Here's how the part is built. I have some questions about the finished solid (model axes, mm). Give positions to 0.01 mm unless a question says otherwise; leave off trailing zeros. Loops run counter-clockwise (first coordinate to the right, second up) from the corner with the lowest first, then second, coordinate; pieces in that order, holes last. Notation, with made-up numbers: (80.25, 12) - (90.25, 12) arc R17 cw to (90.25, 41) - close; hole circle Ø6 at (-6.75, -11). An arc over 180 degrees is marked (long way). Use a Markdown table: item, result.
from build123d import *

# Parameters (mm, degrees)
SKETCH1_R           = 25
BOSS_EXTRUDE1_DEPTH = 3
SKETCH4_R           = 12.5
CUT_EXTRUDE1_DEPTH  = 8.2
SKETCH11_R          = 2
CUT_EXTRUDE2_DEPTH  = 10


with BuildPart() as part:
    # Sketch1 → Boss-Extrude1 (new body)
    with BuildSketch(Plane.XY):
        Circle(SKETCH1_R)
    extrude(amount=BOSS_EXTRUDE1_DEPTH)

    # Sketch4 → Cut-Extrude1 (cut)
    with BuildSketch(Plane(origin=(0, 0, 0), x_dir=(-1, 0, 0), z_dir=(0, 0, -1))):
        Circle(SKETCH4_R)
    extrude(amount=-CUT_EXTRUDE1_DEPTH, mode=Mode.SUBTRACT)

    # Sketch11 → Cut-Extrude2 (cut)
    with BuildSketch(Plane(origin=(0, 0, 0), x_dir=(-1, 0, 0), z_dir=(0, 0, -1))):
        with Locations((0, 18.75)):
            Circle(SKETCH11_R)
        with Locations((16.237976321, 9.375)):
            Circle(SKETCH11_R)
        with Locations((16.237976321, -9.375)):
            Circle(SKETCH11_R)
        with Locations((0, -18.75)):
            Circle(SKETCH11_R)
        with Locations((-16.237976321, -9.375)):
            Circle(SKETCH11_R)
        with Locations((-16.237976321, 9.375)):
            Circle(SKETCH11_R)
    extrude(amount=-CUT_EXTRUDE2_DEPTH, mode=Mode.SUBTRACT)


solid = part.part
(1) Suppose I cut it at C-C on y = -8. Write out the boundary of the cut face in (x, z), plus the area to 3 significant figures.
A:
| item | result |
|---|---|
| outline | (-23.69, 0) - (-17.69, 0) - (-17.69, 3) - (-23.69, 3) - close; (-14.79, 0) - (-9.6, 0) - (-9.6, 3) - (-14.79, 3) - close; (9.6, 0) - (14.79, 0) - (14.79, 3) - (9.6, 3) - close; (17.69, 0) - (23.69, 0) - (23.69, 3) - (17.69, 3) - close |
| area | 67.1 mm2 |
(2) Suppose I cut it at A-A on y = 2. Write out the boundary of the cut face in (x, z).
A:
| item | result |
|---|---|
| outline | (-24.92, 0) - (-12.34, 0) - (-12.34, 3) - (-24.92, 3) - close; (12.34, 0) - (24.92, 0) - (24.92, 3) - (12.34, 3) - close |
(3) Suppose I cut it at D-D on z = 1.8. Write out the boundary of the cut face in (x, y) (3 decimals), plus the area to 3 significant figures.
A:
| item | result |
|---|---|
| outline | circle Ø50 at (0, 0); hole circle Ø4 at (-16.238, -9.375); hole circle Ø4 at (-16.238, 9.375); hole circle Ø25 at (0, 0); hole circle Ø4 at (0, -18.75); hole circle Ø4 at (0, 18.75); hole circle Ø4 at (16.238, -9.375); hole circle Ø4 at (16.238, 9.375) |
| area | 1,400 mm2 |
(4) Suppose I cut it at B-B on x = -4. Write out the boundary of the cut face in (y, z).
A:
| item | result |
|---|---|
| outline | (-24.68, 0) - (-11.84, 0) - (-11.84, 3) - (-24.68, 3) - close; (11.84, 0) - (24.68, 0) - (24.68, 3) - (11.84, 3) - close |
(5) If I drill on line 1 (Y direction, x = 0, z = 1.25); line 2 (Y direction, x = 17, z = 2.25); line 3 (X direction, y = 1, z = 1.25), over which ranges is the centre line in solid material (lowest first)?
A:
| item | result |
|---|---|
| line 1 | -25 to -20.75, -16.75 to -12.5, 12.5 to 16.75, 20.75 to 25 |
| line 2 | -18.33 to -11.22, -7.53 to 7.53, 11.22 to 18.33 |
| line 3 | -24.98 to -12.46, 12.46 to 24.98 |
(6) We'd pull the mould along Y, two halves only. Please class faces 1 (the face through (-5.9, 11.5, 3)), 2 (the face through (23.846, 7.509, 1.479)), 3 (the face through (0.26, 20.733, 1.479)), 4 (the face through (0.26, -16.767, 1.479)): pulls with the +Y half, pulls with the -Y half, needs draft (parallel to the pull), parting line crosses it, or undercut.
A:
| item | result |
|---|---|
| face 1 | needs draft |
| face 2 | parting line crosses it |
| face 3 | undercut |
| face 4 | undercut |
